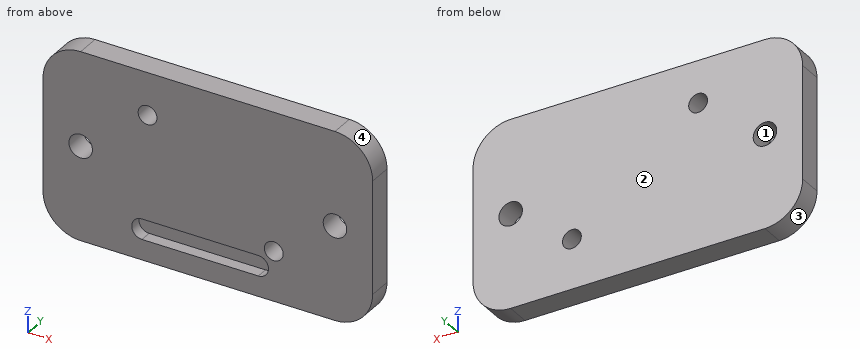
```python
from build123d import *

# Parameters (mm, degrees)
BOSS_EXTRUDE1_DEPTH = 3.175
CUT_EXTRUDE1_REACH  = 5.175
SKETCH2_R           = 1.5875
CUT_EXTRUDE2_REACH  = 5.175
SKETCH3_R           = 1.27
CUT_EXTRUDE3_DEPTH  = 1.5875


with BuildPart() as part:
    # Sketch1 → Boss-Extrude1 (new body)
    with BuildSketch(Plane(origin=(0, 0, 0), x_dir=(1, 0, 0), z_dir=(0, 1, 0))):
        with BuildLine():
            Line((5.08, 0), (39.37, 0))
            ThreePointArc((39.37, 0), (42.962102448, 1.487897552), (44.45, 5.08))
            Line((44.45, 5.08), (44.45, 20.32))
            ThreePointArc((44.45, 20.32), (42.962102448, 23.912102448), (39.37, 25.4))
            Line((39.37, 25.4), (5.08, 25.4))
            ThreePointArc((5.08, 25.4), (1.487897552, 23.912102448), (0, 20.32))
            Line((0, 20.32), (0, 5.08))
            ThreePointArc((0, 5.08), (1.487897552, 1.487897552), (5.08, 0))
        make_face()
    extrude(amount=BOSS_EXTRUDE1_DEPTH)

    # Sketch2 → Cut-Extrude1 (cut, up to next)
    with BuildSketch(Plane.XZ, mode=Mode.PRIVATE) as cut_extrude1_sk1:
        with Locations((5.08, -12.7)):
            Circle(SKETCH2_R)
    cut_extrude1_tool1 = extrude(cut_extrude1_sk1.sketch, amount=-CUT_EXTRUDE1_REACH, mode=Mode.PRIVATE) & part.part
    add(cut_extrude1_tool1.solids().sort_by_distance((5.08, 0, -12.7))[0], mode=Mode.SUBTRACT)
    # Sketch2 → Cut-Extrude1 (cut, up to next)
    with BuildSketch(Plane.XZ, mode=Mode.PRIVATE) as cut_extrude1_sk2:
        with Locations((39.37, -12.7)):
            Circle(SKETCH2_R)
    cut_extrude1_tool2 = extrude(cut_extrude1_sk2.sketch, amount=-CUT_EXTRUDE1_REACH, mode=Mode.PRIVATE) & part.part
    add(cut_extrude1_tool2.solids().sort_by_distance((39.37, 0, -12.7))[0], mode=Mode.SUBTRACT)

    # Sketch3 → Cut-Extrude2 (cut, up to next)
    with BuildSketch(Plane.XZ, mode=Mode.PRIVATE) as cut_extrude2_sk1:
        with Locations((14.097, -5.715)):
            Circle(SKETCH3_R)
    cut_extrude2_tool1 = extrude(cut_extrude2_sk1.sketch, amount=-CUT_EXTRUDE2_REACH, mode=Mode.PRIVATE) & part.part
    add(cut_extrude2_tool1.solids().sort_by_distance((14.097, 0, -5.715))[0], mode=Mode.SUBTRACT)
    # Sketch3 → Cut-Extrude2 (cut, up to next)
    with BuildSketch(Plane.XZ, mode=Mode.PRIVATE) as cut_extrude2_sk2:
        with Locations((31.115, -18.669)):
            Circle(SKETCH3_R)
    cut_extrude2_tool2 = extrude(cut_extrude2_sk2.sketch, amount=-CUT_EXTRUDE2_REACH, mode=Mode.PRIVATE) & part.part
    add(cut_extrude2_tool2.solids().sort_by_distance((31.115, 0, -18.669))[0], mode=Mode.SUBTRACT)

    # Sketch4 → Cut-Extrude3 (cut)
    with BuildSketch(Plane.XZ):
        with BuildLine():
            Line((13.34350835, -19.894123354), (29.031244989, -19.894123354))
            ThreePointArc((29.031244989, -19.894123354), (30.409467748, -21.272346113), (29.031244989, -22.650568872))
            Line((29.031244989, -22.650568872), (13.34350835, -22.650568872))
            ThreePointArc((13.34350835, -22.650568872), (11.965285591, -21.272346113), (13.34350835, -19.894123354))
        make_face()
    extrude(amount=-CUT_EXTRUDE3_DEPTH, mode=Mode.SUBTRACT)


solid = part.part
```
Geometry check sheet. Reference: the model listing, model coordinates, mm. Face numbers are marked on the shaded views. Give positions to 0.01 mm unless a question says otherwise; leave off trailing zeros. Loops run counter-clockwise (first coordinate to the right, second up) from the corner with the lowest first, then second, coordinate; pieces in that order, holes last. Notation, with made-up numbers: (9, 84.25) - (23, 84.25) arc R10 ccw to (23, 90.25) - close; hole circle Ø1 at (72.25, -8). An arc over 180 degrees is marked (long way). Use CSV: the item, a comma, the result in double quotes. Start each with the question number.
Q1. Release check for a two-part mould opening along X. For the marked faces 1, 2, 3 and 4 record: +X half, -X half, draft (parallel to the pull), parting line (faces both ways), or undercut.
Q2. Section check C-C, the plane x = 17.5. Record the cut outline in (y, z) (1 decimal).
Q3. Scan lines: probe 1 along Z at (x, y) = (39.37, 2.1); probe 2 along X at (y, z) = (1.45, -13.75); probe 3 along Z at (x, y) = (28, 1.45). Record each from-to range of solid material in increasing order. Write a range as from..to.
Q4. Section check D-D, the plane z = -22. Record the cut outline in (x, y) (1 decimal), and give its area (3 significant figures).
Q5. Section check A-A, the plane z = -12.7. Count the separate pieces of the cut face and the enclosed holes in it, and give its area (3 significant figures).
Findings below:
1,face 1,"undercut"
1,face 2,"draft"
1,face 3,"-X half"
1,face 4,"+X half"
2,outline,"(0, -25.4) - (3.2, -25.4) - (3.2, 0) - (0, 0) - (0, -19.9) - (1.6, -19.9) - (1.6, -22.7) - (0, -22.7) - close"
3,probe 1,"z = -25.4..-14.29, -11.11..0"
3,probe 2,"x = 0..3.89, 6.27..38.18, 40.56..44.45"
3,probe 3,"z = -25.4..-22.65, -19.89..0"
4,outline,"(0.3, 0) - (12.2, 0) - (12.2, 1.6) - (30.2, 1.6) - (30.2, 0) - (44.2, 0) - (44.2, 3.2) - (0.3, 3.2) - close"
4,area,"111 mm^2"
5,separate pieces,"3"
5,enclosed holes,"0"
5,area,"121 mm^2"
